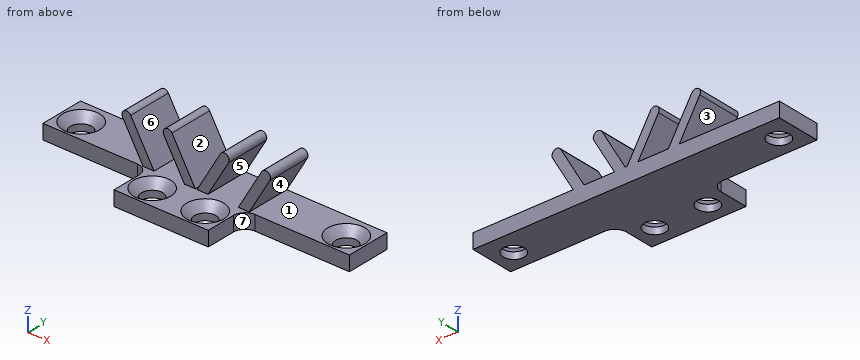
```python
from build123d import *

# Parameters (mm, degrees)
BOSS_EXTRUDE1_DEPTH                                 = 5
SKETCH2_W                                           = 16
SKETCH2_H                                           = 7
SKETCH2_W_2                                         = 7
SKETCH2_H_2                                         = 7.5
CUT_EXTRUDE1_DEPTH                                  = 7.5
CSK_FOR_M3_COUNTERSUNK_FLAT_HEAD_SCREW1_D           = 3.6
CSK_FOR_M3_COUNTERSUNK_FLAT_HEAD_SCREW1_DEPTH       = 5
CSK_FOR_M3_COUNTERSUNK_FLAT_HEAD_SCREW1_CSINK_D     = 6.3
CSK_FOR_M3_COUNTERSUNK_FLAT_HEAD_SCREW1_CSINK_ANGLE = 90
CSK_FOR_M3_COUNTERSUNK_FLAT_HEAD_SCREW1_TIP         = 1.081549114
FILLET1_R                                           = 2
CUT_EXTRUDE2_DEPTH                                  = 7.5


with BuildPart() as part:
    # Sketch1 → Boss-Extrude1 (new, symmetric)
    with BuildSketch(Plane.XY):
        Polygon((26, 7.25), (26, -0.25), (8, -0.25), (8, -7.25), (-8, -7.25), (-8, -0.25), (-26, -0.25), (-26, 7.25), align=None)
    extrude(amount=BOSS_EXTRUDE1_DEPTH, both=True)

    # Sketch2 → Cut-Extrude1 (cut)
    with BuildSketch(Plane.XY.offset(5)):
        with Locations((0, -3.75)):
            Rectangle(SKETCH2_W, SKETCH2_H)
        with Locations((22.5, 3.5)):
            Rectangle(SKETCH2_W_2, SKETCH2_H_2)
        with Locations((-22.5, 3.5)):
            Rectangle(SKETCH2_W_2, SKETCH2_H_2)
    extrude(amount=-CUT_EXTRUDE1_DEPTH, mode=Mode.SUBTRACT)

    # CSK for M3 Countersunk Flat Head Screw1
    with Locations(Plane.XY.offset(-2.5)):
        with Locations((-4.5, -3.75), (4.5, -3.75), (-22.5, 3.25), (22.5, 3.25)):
            CounterSinkHole(CSK_FOR_M3_COUNTERSUNK_FLAT_HEAD_SCREW1_D / 2, CSK_FOR_M3_COUNTERSUNK_FLAT_HEAD_SCREW1_CSINK_D / 2, depth=CSK_FOR_M3_COUNTERSUNK_FLAT_HEAD_SCREW1_DEPTH, counter_sink_angle=CSK_FOR_M3_COUNTERSUNK_FLAT_HEAD_SCREW1_CSINK_ANGLE)
            with Locations((0, 0, -(CSK_FOR_M3_COUNTERSUNK_FLAT_HEAD_SCREW1_DEPTH + CSK_FOR_M3_COUNTERSUNK_FLAT_HEAD_SCREW1_TIP / 2))):  # 118° drill point
                Cone(0, CSK_FOR_M3_COUNTERSUNK_FLAT_HEAD_SCREW1_D / 2, CSK_FOR_M3_COUNTERSUNK_FLAT_HEAD_SCREW1_TIP, mode=Mode.SUBTRACT)

    # Fillet1
    fillet1_edges = [part.edges().sort_by_distance(p)[0] for p in [
        (8, -0.25, -3.75),
        (-8, -0.25, -3.75),
    ]]
    fillet(fillet1_edges, radius=FILLET1_R)

    # Sketch6 → Cut-Extrude2 (cut)
    with BuildSketch(Plane(origin=(0, 7.25, 0), x_dir=(1, 0, 0), z_dir=(0, 1, 0))):
        with BuildLine():
            Line((13.330127019, -5), (11.482606158, -5))
            Line((11.482606158, -5), (4.480127019, -5))
            Line((4.480127019, -5), (-19, -5))
            Line((-19, -5), (-19, 2.5))
            Line((-19, 2.5), (-9, 2.5))
            Line((-9, 2.5), (-12.493246804, -3.550480947))
            ThreePointArc((-12.493246804, -3.550480947), (-12.200426481, -4.64330127), (-11.107606158, -4.350480947))
            Line((-11.107606158, -4.350480947), (-7.152479139, 2.5))
            Line((-7.152479139, 2.5), (-1.997520861, 2.5))
            Line((-1.997520861, 2.5), (-5.490767665, -3.550480947))
            ThreePointArc((-5.490767665, -3.550480947), (-5.197947342, -4.64330127), (-4.105127019, -4.350480947))
            Line((-4.105127019, -4.350480947), (-0.15, 2.5))
            Line((-0.15, 2.5), (0.15, 2.5))
            Line((0.15, 2.5), (4.105127019, -4.350480947))
            ThreePointArc((4.105127019, -4.350480947), (5.197947342, -4.64330127), (5.490767665, -3.550480947))
            Line((5.490767665, -3.550480947), (1.997520861, 2.5))
            Line((1.997520861, 2.5), (7.152479139, 2.5))
            Line((7.152479139, 2.5), (11.107606158, -4.350480947))
            ThreePointArc((11.107606158, -4.350480947), (12.200426481, -4.64330127), (12.493246804, -3.550480947))
            Line((12.493246804, -3.550480947), (9, 2.5))
            Line((9, 2.5), (19, 2.5))
            Line((19, 2.5), (19, -5))
            Line((19, -5), (13.330127019, -5))
        make_face()
    extrude(amount=-CUT_EXTRUDE2_DEPTH, mode=Mode.SUBTRACT)


solid = part.part
```
CAD build for the part. Positions are in the model's coordinates, mm. Face numbers are marked on the shaded views. A direction names the side the tool comes from. Round coordinates to 2 decimals unless told otherwise and drop trailing zeros. Write each loop counter-clockwise with the first axis right and the second up, starting at its lowest first coordinate (ties: lowest second). Pieces come first, ordered by that corner, then holes.
Item 1: Drop flat-ended pins along their axis: pin 1 Ø5 at (x, y) = (9, -0.5) entering from +Z; pin 2 Ø3 at (x, y) = (-7.5, -4.5) entering from +Z; pin 3 Ø2 at (x, z) = (-19, -3.5) entering from -Y; pin 4 Ø2 at (x, y) = (-22.5, 3.25) entering from +Z. Give the stop position or say it passes through.
Filled in:
pin 1: stops at z = 4.69
pin 2: stops at z = -2.5
pin 3: stops at y = -0.25
pin 4: passes through
Item 2: Band-saw the part on C-C on z = -1.25. Write the cut outline in (x, y).
Filled in:
outline: (-9.72, -0.25) - (-7.87, -0.25) - (-7.87, 7.25) - (-9.72, 7.25) - close; (-2.72, -0.25) - (-0.87, -0.25) - (-0.87, 7.25) - (-2.72, 7.25) - close; (0.87, -0.25) - (2.72, -0.25) - (2.72, 7.25) - (0.87, 7.25) - close; (7.87, -0.25) - (9.72, -0.25) - (9.72, 7.25) - (7.87, 7.25) - close
Item 3: Drill centre lines: L1, parallel to X at y = 3.25, z = -4.05; L2, parallel to X at y = -3.75, z = -4.25; L3, parallel to Y at x = 22.5, z = -4.15. Where is each one in solid material? Low to high.
Filled in:
L1: x = -26 to -24.3, -20.7 to 20.7, 24.3 to 26
L2: x = -8 to -6.3, -2.7 to 2.7, 6.3 to 8
L3: y = -0.25 to 1.45, 5.05 to 7.25
Item 4: Band-saw the part on A-A on y = 3.25. Give the number of separate pieces and of enclosed holes in the cut face, then the cut area to 3 significant figures.
Filled in:
separate pieces: 3
enclosed holes: 0
area: 160 mm2
Item 5: Mould opens along X. For the marked faces 1, 2, 3 and 4 say: released by +X, released by -X, zero draft, split by the parting line, or undercut.
Filled in:
face 1: undercut
face 2: undercut
face 3: released by -X
face 4: released by +X
Item 6: Band-saw the part on B-B on x = 22.5. Write the cut outline in (y, z).
Filled in:
outline: (-0.25, -5) - (1.45, -5) - (1.45, -3.85) - (0.1, -2.5) - (-0.25, -2.5) - close; (5.05, -5) - (7.25, -5) - (7.25, -2.5) - (6.4, -2.5) - (5.05, -3.85) - close
Item 7: Band-saw the part on D-D on y = -3.75. Write the cut outline in (x, z).
Filled in:
outline: (-8, -5) - (-6.3, -5) - (-6.3, -3.85) - (-7.65, -2.5) - (-8, -2.5) - close; (-2.7, -5) - (2.7, -5) - (2.7, -3.85) - (1.35, -2.5) - (-1.35, -2.5) - (-2.7, -3.85) - close; (6.3, -5) - (8, -5) - (8, -2.5) - (7.65, -2.5) - (6.3, -3.85) - close
Item 8: Tool access for the marked faces 5, 6 and 7: list every direction of +Z, -Z, +X, -X, +Y, -Y with a clear straight run to the whole face (end or side of a thin tool).
Filled in:
face 5: +Y, -Y
face 6: +Z, +Y, -Y
face 7: +Z, -Z, +X, -Y
